Check sheet for the modelled part. Datum: model origin and axes. Units: mm. A direction names the side the tool comes from. Round coordinates to 2 decimals unless told otherwise and drop trailing zeros. Order: outer loops, then holes, each group sorted by start corner. A loop starts at its lowest first (then second) coordinate and runs counter-clockwise, first axis right, second up. Notation, with made-up numbers: (-11.75, -12) -> (6.25, -12) arc R15 cw to (6.25, 6) -> close; hole circle Ø3 at (49, 20.5). An arc over 180 degrees is marked (long way). Answer in a Markdown table with one row per item.
Autodesk Fusion 360 part; units mm, degrees
sketch "스케치1" plane through (0, 0, 0) normal (0, 1, 0) x (1, 0, 0)
  line L0 (0, 0) -> (0, -30)
  line L1 (0, -30) -> (-16.6337, -53.7554)
  line L2 (0, -30) -> (29, -30) construction
  line L3 (0, 0) -> (-2, 0)
  line L4 (-16.6337, -53.7554) -> (-18.272, -52.6083)
  line L5 (-18.272, -52.6083) -> (-2, -29.3694)
  line L6 (-2, 0) -> (-2, -29.3694)
  line L7 (0, 0) -> (-73, 0)
  line L8 (-16.6337, -53.7554) -> (-73, -53.7554)
  line L9 (-18.272, -52.6083) -> (-17.1249, -50.97)
  line L10 (-73, -53.7554) -> (-73, -48.7554)
  line L11 (-73, -48.7554) -> (-53, -48.7554)
  line L12 (-53, -48.7554) -> (-53, -53.7554)
  line L13 (-17.1249, -50.97) -> (-53, -50.97)
  line L14 (-53, -50.97) -> (-45, -50.97)
  line L15 (-45, -50.97) -> (-45, 0)
  dimension "d1" = 30
  dimension "d2" = 125
  dimension "d3" = 29
  dimension "d4" = 2
  dimension "d7" = 73
  dimension "d8" = 2
  dimension "d9" = 5
  dimension "d10" = 20
  dimension "d11" = 8
extrude "돌출1" add sketch "스케치1" along normal blind 88.975 contours L0 L1 L3 L4 L5 L6 L7 L9 | L4 L5 L8 L9 L12 L13 L14 | L8 L10 L11 L12
extrude "돌출2" add sketch "스케치1" along normal blind 3 contours L5 L6 L7 L13 L15
sketch "스케치2" plane through (0, 88.975, 0) normal (0, 1, 0) x (-1, 0, 0)
  line L0 (0, 0) -> (2, 0)
  line L1 (2, 0) -> (2, 29.3694)
  line L2 (2, 29.3694) -> (17.1249, 50.97)
  line L3 (17.1249, 50.97) -> (53, 50.97)
  line L4 (53, 50.97) -> (53, 48.7554)
  line L5 (53, 48.7554) -> (73, 48.7554)
  line L6 (73, 48.7554) -> (73, 53.7554)
  line L7 (73, 53.7554) -> (16.6337, 53.7554)
  line L8 (16.6337, 53.7554) -> (0, 30)
  line L9 (0, 30) -> (0, 0)
  line L10 (53, 50.97) -> (45, 50.97)
  line L11 (45, 50.97) -> (45, 0)
  line L12 (45, 0) -> (2, 0)
  dimension "d14" = 8
extrude "돌출3" add sketch "스케치2" against normal blind 3 contours L1 L2 L3 L11 L12
sketch "스케치3" plane through (0, 0, 0) normal (1, 0, 0) x (0, 1, 0)
  line L0 (0, 30) -> (0, 0)
  line L1 (0, 0) -> (88.975, 0)
  line L2 (88.975, 0) -> (88.975, 30)
  line L3 (88.975, 30) -> (0, 30)
  line L4 (86.4875, 30) -> (2.4875, 30)
  line L5 (2.4875, 30) -> (2.4875, 0)
  line L6 (2.4875, 0) -> (86.4875, 0)
  line L7 (86.4875, 0) -> (86.4875, 30)
  line L8 (86.4875, 30) -> (2.4875, 0) construction
  line L9 (2.4875, 30) -> (86.4875, 0) construction
  line L10 (2.4875, 15) -> (16.4875, 15)
  line L11 (16.4875, 15) -> (30.4875, 15)
  line L12 (30.4875, 15) -> (44.4875, 15)
  line L13 (44.4875, 15) -> (58.4875, 15)
  line L14 (58.4875, 15) -> (74.4875, 15)
  line L15 (74.4875, 15) -> (86.4875, 15)
  circle A0 centre (16.4875, 15) radius 3.25
  circle A1 centre (30.4875, 15) radius 3.25
  circle A2 centre (44.4875, 15) radius 3.25
  circle A3 centre (58.4875, 15) radius 3.25
  circle A4 centre (74.4875, 15) radius 6
  circle A5 centre (16.4875, 15) radius 6
  point P0 (44.4875, 15)
  dimension "d45" = 84
  dimension "d46" = 14
  dimension "d47" = 14
  dimension "d48" = 14
  dimension "d49" = 14
  dimension "d50" = 16
  dimension "d51" = 6.5
  dimension "d52" = 6.5
  dimension "d53" = 6.5
  dimension "d54" = 6.5
  dimension "d55" = 12
  dimension "d56" = 12
extrude "돌출4" cut sketch "스케치3" against normal blind 3 contours L14 L15 A4 | L14 L15 A4 | L10 L11 A0 | L10 L11 A0 | L11 L12 A1 | L11 L12 A1 | L13 L14 A3 | L13 L14 A3 | L12 L13 A2 | L12 L13 A2
sketch "스케치4" plane through (14.0954, 0, 9.8697) normal (0.8192, 0, 0.5736) x (0, 1, 0)
  line L0 (0, 53.5746) -> (0, 24.5746)
  line L1 (0, 24.5746) -> (88.975, 24.5746)
  line L2 (88.975, 24.5746) -> (88.975, 53.5746)
  line L3 (88.975, 53.5746) -> (0, 53.5746)
  line L4 (0, 39.0746) -> (32.5, 39.0746)
  line L5 (7.4, 28.9746) -> (57.6, 28.9746)
  line L6 (57.6, 28.9746) -> (57.6, 49.1746)
  line L7 (57.6, 49.1746) -> (7.4, 49.1746)
  line L8 (7.4, 49.1746) -> (7.4, 28.9746)
  line L9 (7.4, 28.9746) -> (57.6, 49.1746) construction
  line L10 (57.6, 28.9746) -> (7.4, 49.1746) construction
  line L11 (88.975, 39.0746) -> (75, 39.0746)
  line L12 (68.525, 49.0746) -> (81.475, 49.0746)
  line L13 (81.475, 49.0746) -> (81.475, 29.0746)
  line L14 (81.475, 29.0746) -> (68.525, 29.0746)
  line L15 (68.525, 29.0746) -> (68.525, 49.0746)
  line L16 (68.525, 49.0746) -> (81.475, 29.0746) construction
  line L17 (81.475, 49.0746) -> (68.525, 29.0746) construction
  point P0 (32.5, 39.0746)
  point P1 (75, 39.0746)
  dimension "d37" = 32.5
  dimension "d38" = 50.2
  dimension "d39" = 20.2
  dimension "d40" = 13.975
  dimension "d41" = 12.95
  dimension "d42" = 20
extrude "돌출5" cut sketch "스케치4" against normal blind 3 contours L5 L6 L7 L8 | L12 L13 L14 L15
sketch "스케치5" plane through (0, 88.975, 0) normal (0, 1, 0) x (-1, 0, 0)
  line L0 (0, 0) -> (45, 0)
  line L1 (45, 0) -> (45, 50.97)
  line L2 (45, 50.97) -> (53, 50.97)
  line L3 (53, 50.97) -> (53, 48.7554)
  line L4 (53, 48.7554) -> (73, 48.7554)
  line L5 (73, 48.7554) -> (73, 53.7554)
  line L6 (73, 53.7554) -> (16.6337, 53.7554)
  line L7 (16.6337, 53.7554) -> (0, 30)
  line L8 (0, 30) -> (0, 0)
  line L9 (0, 30) -> (5, 30)
  line L10 (5, 0) -> (5, 5)
  line L11 (5, 5) -> (5, 30)
  line L12 (5, 5) -> (40, 5)
  line L13 (5, 30) -> (21.6337, 53.7554)
  line L14 (5, 30) -> (5, 25)
  line L15 (5, 25) -> (45, 25)
  line L16 (45, 53.7554) -> (45, 48.7554)
  line L17 (45, 48.7554) -> (28.3663, 25)
  line L18 (28.3663, 25) -> (28.3663, 0)
  line L19 (28.3663, 5) -> (33.3663, 5)
  line L20 (33.3663, 5) -> (33.3663, 0)
  line L21 (33.3663, 5) -> (33.3663, 25)
  line L22 (45, 48.7554) -> (50, 48.7554)
  line L23 (50, 48.7554) -> (33.3663, 25)
  line L24 (45, 48.7554) -> (18.1327, 48.7554)
  line L25 (45, 53.7554) -> (40, 53.7554)
  line L26 (40, 53.7554) -> (40, 34.4739)
  line L27 (40, 34.4739) -> (45, 34.4739)
  line L28 (45, 34.4739) -> (45, 53.7554)
  line L29 (33.3663, 5) -> (28.3663, 0)
  dimension "d57" = 5
  dimension "d58" = 5
  dimension "d59" = 35
  dimension "d60" = 29
  dimension "d61" = 5
  dimension "d62" = 5
  dimension "d63" = 29
  dimension "d64" = 5
  dimension "d65" = 5
  dimension "d66" = 5
extrude "돌출6" cut sketch "스케치5" against normal blind 88.975 contours L0 L20 L29 | L11 L12 L15 L18 | L11 L13 L14 L15 L17 L24 L26 | L0 L1 L15 L20 L21 | L1 L15 L23 L27 | L1 L23 L27 L28
sketch "스케치6" plane through (0, 0, 53.7554) normal (0, 0, 1) x (-1, 0, 0)
  line L0 (73, 0) -> (16.6337, 0)
  line L1 (16.6337, 0) -> (16.6337, -88.975)
  line L2 (16.6337, -88.975) -> (73, -88.975)
  line L3 (73, -88.975) -> (73, 0)
  line L4 (73, 0) -> (53, 0)
  line L5 (53, 0) -> (53, -88.975)
  line L6 (53, -88.975) -> (73, -88.975)
  line L7 (73, -88.975) -> (73, 0)
  line L8 (73, 0) -> (53, 0)
  line L9 (53, 0) -> (53, -20)
  line L10 (53, -20) -> (73, -20)
  line L11 (73, -20) -> (73, 0)
  line L12 (73, -88.975) -> (53, -88.975)
  line L13 (53, -88.975) -> (53, -68.975)
  line L14 (53, -68.975) -> (73, -68.975)
  line L15 (73, -68.975) -> (73, -88.975)
  circle A0 centre (63, -10) radius 2.65
  circle A1 centre (63, -78.975) radius 2.65
  dimension "d69" = 20
  dimension "d70" = 20
  dimension "d71" = 20
  dimension "d72" = 5.3
  dimension "d73" = 5.3
extrude "돌출7" cut sketch "스케치6" against normal blind 5 contours L3 L5 L7 L10 L14 | A0 | A1
(1) Depth check by flat-ended pin: pin 1 Ø1.5 at (y, z) = (2, 43.5) entering from +X; pin 2 Ø2.5 at (x, y) = (-34.5, 1.5) entering from -Z; pin 3 Ø8 at (y, z) = (26, 35) entering from -X. Enter the tip coordinate at first touch or a pass-through.
Solutions:
| item | result |
|---|---|
| pin 1 | x = -8.93 |
| pin 2 | z = 4.88 |
| pin 3 | x = -4.16 |
(2) Section check B-B on x = -63. Record the boundary of the cut face in (y, z) (3 decimals).
Solutions:
| item | result |
|---|---|
| outline | (0, 48.755) -> (7.35, 48.755) -> (7.35, 53.755) -> (0, 53.755) -> close; (12.65, 48.755) -> (20, 48.755) -> (20, 53.755) -> (12.65, 53.755) -> close; (68.975, 48.755) -> (76.325, 48.755) -> (76.325, 53.755) -> (68.975, 53.755) -> close; (81.625, 48.755) -> (88.975, 48.755) -> (88.975, 53.755) -> (81.625, 53.755) -> close |
(3) Tool access check on faces 1 (the flat face through (-53, 79, 50)), 2 (the flat face through (-53, 44, 52)), 3 (the flat face through (-34.26, 1.52, 33.42)). Record the directions out of +Z, -Z, +X, -X, +Y, -Y that give a thin tool (end or side, any length) a straight path to the whole face; none if there is none.
Solutions:
| item | result |
|---|---|
| face 1 | -Z, +Y, -Y |
| face 2 | +Z, -Z, -X |
| face 3 | +Y, -Y |
(4) Section check A-A on y = 37. Record the boundary of the cut face in (x, z).
Solutions:
| item | result |
|---|---|
| outline | (-53, 50.97) -> (-17.12, 50.97) -> (-15.75, 49) -> (-14.11, 50.15) -> (-16.63, 53.76) -> (-53, 53.76) -> close; (-4.16, 32.46) -> (-2, 29.37) -> (-2, 0) -> (0, 0) -> (0, 30) -> (-2.52, 33.6) -> close |
(5) Draft check along X on faces 4 (the flat face through (-33.366, 87, 15)), 5 (the flat face through (-9, 81.475, 41)), 6 (the flat face through (-5, 87, 17)). Enter one of: pulls with the +X half, pulls with the -X half, needs draft (parallel to the pull), parting line crosses it, or undercut.
Solutions:
| item | result |
|---|---|
| face 4 | pulls with the -X half |
| face 5 | needs draft |
| face 6 | undercut |
(6) Scan lines: probe 1 along Y at (x, z) = (-63, 52) (3 decimals); probe 2 along Y at (x, z) = (-1.1, 15) (1 decimal); probe 3 along Y at (x, z) = (-32.5, 22.5) (3 decimals). Record each from-to range of solid material in increasing order. Write a range as from..to.
Solutions:
| item | result |
|---|---|
| probe 1 | 0..7.35, 12.65..20, 68.975..76.325, 81.625..88.975 |
| probe 2 | 0..13.2, 19.7..27.2, 33.7..41.2, 47.7..55.2, 61.7..68.5, 80.5..89 |
| probe 3 | 0..3, 85.975..88.975 |
(7) Section check C-C on z = 26.5. Record the boundary of the cut face in (x, y) (3 decimals).
Solutions:
| item | result |
|---|---|
| outline | (-34.417, 0) -> (-29.417, 0) -> (-29.417, 3) -> (-34.417, 3) -> close; (-34.417, 85.975) -> (-29.417, 85.975) -> (-29.417, 88.975) -> (-34.417, 88.975) -> close; (-5, 0) -> (0, 0) -> (0, 88.975) -> (-5, 88.975) -> (-5, 85.975) -> (-2, 85.975) -> (-2, 3) -> (-5, 3) -> close |
(8) Section check D-D on y = 10. Record the boundary of the cut face in (x, z), plus the area to 3 significant figures.
Solutions:
| item | result |
|---|---|
| outline | (-73, 48.76) -> (-65.65, 48.76) -> (-65.65, 53.76) -> (-73, 53.76) -> close; (-60.35, 48.76) -> (-53, 48.76) -> (-53, 50.97) -> (-17.12, 50.97) -> (-15.75, 49) -> (-14.11, 50.15) -> (-16.63, 53.76) -> (-60.35, 53.76) -> close; (-4.16, 32.46) -> (-2, 29.37) -> (-2, 0) -> (0, 0) -> (0, 30) -> (-2.52, 33.6) -> close |
| area | 248 mm^2 |
